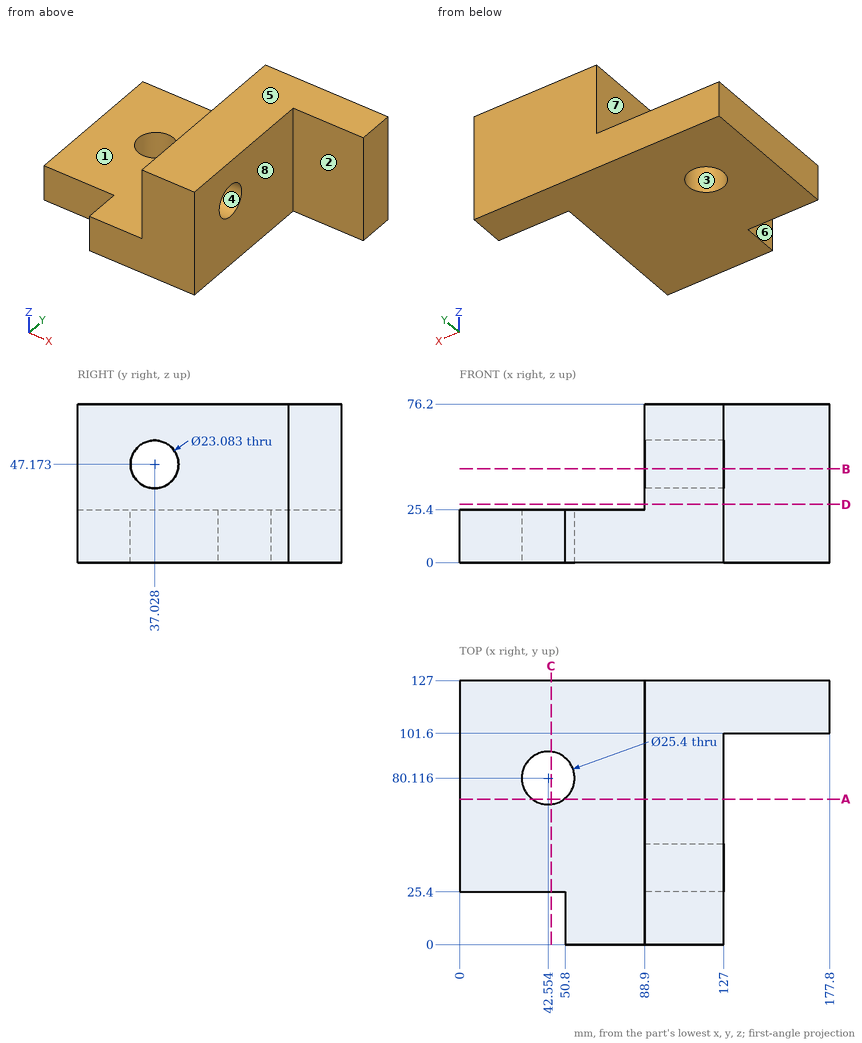
Verification items for this drawing (mm, ordinates from the low corner). A direction names the side the tool comes from. Give positions to 0.01 mm unless a question says otherwise; leave off trailing zeros. Loops run counter-clockwise (first coordinate to the right, second up) from the corner with the lowest first, then second, coordinate; pieces in that order, holes last. Notation, with made-up numbers: M 72.5,8.25 L 96.5,8.25 A22 cw 96.5,20.25 Z; hole C 27.5,22 d1. An arc over 180 degrees is marked long. Write item = value, one per line. Start each with the question number.
1. Go/stop test with flat-tipped pins: P1, Ø2, axis at x = 30.5, y = 27, coming from the +Z side; P2, Ø5, axis at y = 17, z = 46.5, coming from the -X side; P3, Ø12.5, axis at y = 9, z = 16, coming from the -X side. Record where each tip stops, or that it passes through.
2. Draft check along Y on the marked faces 1, 2, 3 and 4. Enter one of: +Y half, -Y half, draft (parallel to the pull), parting line (faces both ways), or undercut.
3. Section check B-B, the plane z = 45. Enter the section's corners in (x, y).
4. Tool access check on the marked faces 5, 6, 7 and 8. Record the directions out of +Z, -Z, +X, -X, +Y, -Y that give a thin tool (end or side, any length) a straight path to the whole face; none if there is none.
5. Section check A-A, the plane y = 70. Enter the section's corners in (x, z), plus the area to 3 significant figures.
6. Section check D-D, the plane z = 28. Enter the section's corners in (x, y).
7. Section check C-C, the plane x = 44. Enter the section's corners in (y, z).
8. Thickness scan on probe 1 along Z at (x, y) = (81.5, 50.5); probe 2 along X at (y, z) = (52.5, 30); probe 3 along X at (y, z) = (14, 21). Record the ranges inside material, lowest first.
Values follow:
q1.P1 = 25.4
q1.P2 = 88.9
q1.P3 = 50.8
q2.face_1 = draft
q2.face_2 = -Y half
q2.face_3 = undercut
q2.face_4 = undercut
q3.outline = M 88.9,0 L 127,0 L 127,25.69 L 88.9,25.69 Z; M 88.9,48.36 L 127,48.36 L 127,101.6 L 177.8,101.6 L 177.8,127 L 88.9,127 Z
q4.face_5 = +Z, +X, -X, +Y, -Y
q4.face_6 = +Z, -Z, -X, -Y
q4.face_7 = +Z, -X, +Y, -Y
q4.face_8 = +Z, -Z, +X, -Y
q5.outline = M 0,0 L 34.88,0 L 34.88,25.4 L 0,25.4 Z; M 50.23,0 L 127,0 L 127,76.2 L 88.9,76.2 L 88.9,25.4 L 50.23,25.4 Z
q5.area = 4,770 mm^2
q6.outline = M 88.9,0 L 127,0 L 127,101.6 L 177.8,101.6 L 177.8,127 L 88.9,127 Z
q7.outline = M 25.4,0 L 67.5,0 L 67.5,25.4 L 25.4,25.4 Z; M 92.73,0 L 127,0 L 127,25.4 L 92.73,25.4 Z
q8.probe_1 = 0 to 25.4
q8.probe_2 = 88.9 to 127
q8.probe_3 = 50.8 to 127
